Part model, mm, in its own coordinate system. A direction names the side the tool comes from. Give positions to 0.01 mm unless a question says otherwise; leave off trailing zeros. Write each loop counter-clockwise with the first axis right and the second up, starting at its lowest first coordinate (ties: lowest second). Pieces come first, ordered by that corner, then holes. Notation, with made-up numbers: M -24.5,22.5 L 5.5,22.5 A15 ccw 5.5,30.5 Z; hole C -15,39 d8. An arc over 180 degrees is marked long. Use a Markdown table: item, result. Add a question column.
Autodesk Inventor part; units mm, degrees
ref_plane "YZ Plane" through (0, 0, 0) normal (1, 0, 0) x (0, 1, 0)
ref_plane "XZ Plane" through (0, 0, 0) normal (0, 1, 0) x (-1, 0, 0)
ref_plane "XY Plane" through (0, 0, 0) normal (0, 0, 1) x (1, 0, 0)
sketch "Sketch1" plane through (0, 0, 0) normal (0, 1, 0) x (-1, 0, 0)
  circle A0 centre (0, 0) radius 16.25
  dimension "d0" = 32.5
extrude "Extrusion1" add sketch "Sketch1" along normal blind 40
chamfer "Chamfer1" distance 4 angle 45 1 edges at (16.25, 0, 0)
sketch "Sketch2" plane through (0, 40, 0) normal (0, 1, 0) x (1, 0, 0)
  circle A0 centre (0, 0) radius 12
  circle A1 centre (0, 0) radius 16.25
  dimension "d6" = 24
extrude "Extrusion2" cut sketch "Sketch2" against normal blind 30
sketch "Sketch3" plane through (0, 0, 0) normal (0, -1, 0) x (1, 0, 0)
  circle A0 centre (0, 0) radius 12
extrude "Extrusion3" cut sketch "Sketch3" against normal blind 2
sketch "Sketch4" plane through (0, 2, 0) normal (0, -1, 0) x (1, 0, 0)
  circle A0 centre (0, 0) radius 11.5
  dimension "d11" = 23
extrude "Extrusion4" add sketch "Sketch4" along normal blind 4
fillet "Fillet1" radius 2 1 edges at (-11.5, -2, 0)
properties part number "Buton_1"
1. Cut at C-C (y = 29). Write the cut outline in (x, z), then the cut area to 3 significant figures.
2. Drill centre lines: probe 1 along Z at (x, y) = (0, 1); probe 2 along Z at (x, y) = (0, 0.6); probe 3 along X at (y, z) = (0.5, -3). Where is each one in solid material? Low to high. Write a range as [from, to].
3. Mould opens along Z. For faces 3 (the cylindrical face through (-1.5, 1, -11.4)), 4 (the cylindrical face through (-11.99, 25.21, -0.53)), 5 (the flat face through (6, 2, -10)), 6 (the flat face through (-7, 10, 10)) say: released by +Z, released by -Z, zero draft, split by the parting line, or undercut.
4. Cut at B-B (x = 0). Write the cut outline in (y, z).
5. Cut at A-A (z = 0). Write the cut outline in (x, y).
6. Flat gauge pins, fed straight in: pin 1 (1 mm diameter, centred on x = -11, z = 4, fed in from -Y); pin 2 (1 mm diameter, centred on x = 3.5, z = -13, fed in from -Y); pin 3 (5 mm diameter, centred on x = -7.5, y = 10, fed in from +Z). Where does each tip first touch, or does it go through?
7. Tool access for faces 1 (the cylindrical face through (-11.99, 0.99, 0.53)), 2 (the flat face through (0, 40, 0)): list every direction of +Z, -Z, +X, -X, +Y, -Y with a clear straight run to the whole face (end or side of a thin tool).
A:
| question | item | result |
|---|---|---|
| 1 | outline | C 0,0 d24 |
| 1 | area | 452 mm² |
| 2 | probe 1 | z = [-13.25, -12], [-11.5, 11.5], [12, 13.25] |
| 2 | probe 2 | z = [-12.85, -12], [-11.5, 11.5], [12, 12.85] |
| 2 | probe 3 | x = [-12.39, -11.62], [-11.1, 11.1], [11.62, 12.39] |
| 3 | face 3 | undercut |
| 3 | face 4 | split by the parting line |
| 3 | face 5 | undercut |
| 3 | face 6 | zero draft |
| 4 | outline | M -2,-9.5 A2 ccw 0,-11.5 L 2,-11.5 L 2,-12 L 0,-12 L 0,-12.25 L 4,-16.25 L 10,-16.25 L 10,-12 L 40,-12 L 40,12 L 10,12 L 10,16.25 L 4,16.25 L 0,12.25 L 0,12 L 2,12 L 2,11.5 L 0,11.5 A2 ccw -2,9.5 Z |
| 5 | outline | M -16.25,4 L -12.25,0 L -12,0 L -12,2 L -11.5,2 L -11.5,0 A2 ccw -9.5,-2 L 9.5,-2 A2 ccw 11.5,0 L 11.5,2 L 12,2 L 12,0 L 12.25,0 L 16.25,4 L 16.25,10 L 12,10 L 12,40 L -12,40 L -12,10 L -16.25,10 Z |
| 6 | pin 1 | stops at y = -1.05 |
| 6 | pin 2 | stops at y = 0.71 |
| 6 | pin 3 | stops at z = 15.46 |
| 7 | face 1 | -Y |
| 7 | face 2 | +Z, -Z, +X, -X, +Y |
